```python
from build123d import *

# Parameters (mm, degrees)
F0_R           = 12.7
F1_DEPTH       = 7.9
F1_FACE_R      = 12.7
F2_DEPTH       = 3
F3_DEPTH       = 3
F4_R           = 5
F8_D           = 3.3
F8_CBORE_D     = 6
F8_CBORE_DEPTH = 3.3


# Not quite as in the source:
# - a feature names something its author has since deleted; it is built from what else it names


with BuildPart() as f1:
    # F0 (on Top) → F1 (new body)
    with BuildSketch(Plane.XY):
        with BuildLine():
            ThreePointArc((-82.519158721, -19.8666825891), (-82.3199649398, 11.4193737584), (-65.6162592679, 37.8739237785))
            Line((-65.6162592679, 37.8739237785), (-99.2088739193, 37.8739237785))
            ThreePointArc((-99.2088739193, 37.8739237785), (-117.1879721114, 26.6373104948), (-114.9666717313, 5.5523567478))
            Line((-114.9666717313, 5.5523567478), (-81.4747432756, -37.2867286205))
            Line((-81.4747432756, -37.2867286205), (-73.9695476283, -37.2867286205))
            Line((-73.9695476283, -37.2867286205), (-82.519158721, -19.8666825891))
        make_face()
        with Locations((-99.2088739193, 17.8719250206)):
            Circle(F0_R, mode=Mode.SUBTRACT)
    extrude(amount=-F1_DEPTH)



with BuildPart() as f1b:
    # F0 (on Top) → F1, piece 2 (new body)
    with BuildSketch(Plane.XY):
        with BuildLine():
            Line((86, -37.2867286205), (86, 37.8739237785))
            ThreePointArc((86, 37.8739237785), (76.5230858808, 21.4851908555), (70.8448413014, 3.4252903424))
            ThreePointArc((70.8448413014, 3.4252903424), (70.5487291916, -0.5692843065), (71.2877699379, -4.5060504646))
            ThreePointArc((71.2877699379, -4.5060504646), (77.4631412951, -21.4263167299), (86, -37.2867286205))
        make_face()
    extrude(amount=-F1_DEPTH)


with BuildPart() as f1_1:
    add(f1.part)

    add(f1b.part)  # F2 merges F1b
    # F0 (on Top) + F1_face (on face) → F2 (join)
    with BuildSketch(Plane.XY):
        with BuildLine():
            ThreePointArc((70.8448413014, 3.4252903424), (76.5230858808, 21.4851908555), (86, 37.8739237785))
            Line((86, 37.8739237785), (-65.6162592679, 37.8739237785))
            ThreePointArc((-65.6162592679, 37.8739237785), (-82.3199649398, 11.4193737584), (-82.519158721, -19.8666825891))
            Line((-82.519158721, -19.8666825891), (-73.9695476283, -37.2867286205))
            Line((-73.9695476283, -37.2867286205), (86, -37.2867286205))
            ThreePointArc((86, -37.2867286205), (77.4631412951, -21.4263167299), (71.2877699379, -4.5060504646))
            ThreePointArc((71.2877699379, -4.5060504646), (70.5487291916, -0.5692843065), (70.8448413014, 3.4252903424))
        make_face()
    with BuildSketch(Plane(origin=(-93.510683798, 7.7887517246, 0), x_dir=(1, 0, 0), z_dir=(0, 0, 1))):
        with BuildLine():
            ThreePointArc((10.9915250771, -27.6554343137), (11.1907188583, 3.6306220338), (27.8944245301, 30.0851720539))
            Line((27.8944245301, 30.0851720539), (-5.6981901212, 30.0851720539))
            ThreePointArc((-5.6981901212, 30.0851720539), (-23.6772883134, 18.8485587701), (-21.4559879333, -2.2363949769))
            Line((-21.4559879333, -2.2363949769), (12.0359405224, -45.0754803451))
            Line((12.0359405224, -45.0754803451), (19.5411361698, -45.0754803451))
            Line((19.5411361698, -45.0754803451), (10.9915250771, -27.6554343137))
        make_face()
        with Locations((-5.6981901212, 10.083173296)):
            Circle(F1_FACE_R, mode=Mode.SUBTRACT)
    extrude(amount=F2_DEPTH)

    # F4
    f4_edges = [f1_1.edges().sort_by_distance(p)[0] for p in [
        (-81.474743, -37.286729, -2.45),
    ]]
    fillet(f4_edges, radius=F4_R)


with BuildPart() as f3:
    # F0 (on Top) → F3 (new body)
    with BuildSketch(Plane.XY):
        with BuildLine():
            Line((86, -37.2867286205), (86, 37.8739237785))
            ThreePointArc((86, 37.8739237785), (76.5230858808, 21.4851908555), (70.8448413014, 3.4252903424))
            ThreePointArc((70.8448413014, 3.4252903424), (70.5487291916, -0.5692843065), (71.2877699379, -4.5060504646))
            ThreePointArc((71.2877699379, -4.5060504646), (77.4631412951, -21.4263167299), (86, -37.2867286205))
        make_face()
    extrude(amount=F3_DEPTH)


with BuildPart() as f1_2:
    add(f1_1.part)

    # F6: union F3
    add(f3.part)

    # F8 (through all)
    with Locations(Plane.XY.offset(3)):
        with Locations((-76.3588739193, 33.2139237785), (-113.9428039086, 24.5539237785), (-81.1954878403, -31.5067286205), (82.39, -23.6667286205), (82.39, 25.7039237785)):
            CounterBoreHole(F8_D / 2, F8_CBORE_D / 2, F8_CBORE_DEPTH)


solid = f1_2.part
```
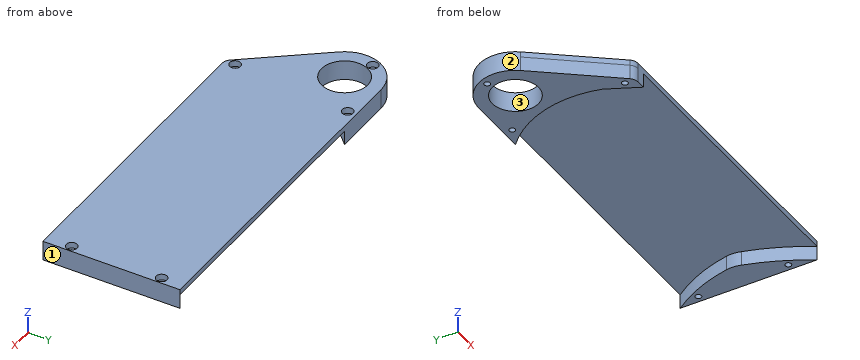
Geometry: final body of the model. Coordinates: model frame, mm. Face numbers are marked on the shaded views. Give positions to 0.01 mm unless a question says otherwise; leave off trailing zeros. Loops run counter-clockwise (first coordinate to the right, second up) from the corner with the lowest first, then second, coordinate; pieces in that order, holes last. Notation, with made-up numbers: (39, 89) - (45, 89) arc R21 ccw to (45, 103) - close; hole circle Ø9 at (32, 30.25). An arc over 180 degrees is marked (long way). Answer as CSV lines item,"result". Start each with the question number.
(1) Mould query, pull axis Y, two halves, no side actions, for the marked faces 1, 2 and 3. Classes: +Y half, -Y half, draft (parallel to the pull), parting line (faces both ways), or undercut.
(2) Section query C-C (y = -13). Output: boundary loops of the cut face in (x, z).
(3) Section query B-B (y = 14.5). Output: boundary loops of the cut face in (x, z), and give its area (3 significant figures).
(4) Ray query, line 1 along X through (y, z) = (15.5, -6.5); line 2 along Z through (x, y) = (-56.5, 22.5); line 3 along X through (y, z) = (-22.5, -1). Return the intervals inside material, ascending. Write a range as [from, to].
(5) Section query A-A (z = -5). Output: boundary loops of the cut face in (x, y).
(6) Pin query (flat end, axial travel): P1, Ø1.5, axis at y = -5.5, z = -4, coming from the -X side; P2, Ø1.8, axis at x = -80.5, y = -33, coming from the +Z side; P3, Ø1.5, axis at y = 24.5, z = -2.5, coming from the -X side. Return the tip coordinate at first contact, or that it passes through.
(7) Section query D-D (x = -58.5). Output: boundary loops of the cut face in (y, z), and give its area (3 significant figures).
Worked answers:
1,face 1,"draft"
1,face 2,"parting line"
1,face 3,"undercut"
2,outline,"(-100.46, -7.9) - (-83.99, -7.9) - (-83.99, 0) - (74.04, 0) - (74.04, -7.9) - (86, -7.9) - (86, 3) - (-100.46, 3) - close"
3,outline,"(-118.92, -7.9) - (-111.45, -7.9) - (-111.45, 3) - (-118.92, 3) - close; (-86.96, -7.9) - (-81.32, -7.9) - (-81.32, 0) - (73.81, 0) - (73.81, -7.9) - (86, -7.9) - (86, 3) - (-86.96, 3) - close"
3,area,"741 mm^2"
4,line 1,"x = [-119.07, -111.69], [-86.73, -80.96], [74.15, 86]"
4,line 2,"z = [0, 3]"
4,line 3,"x = [-93.04, -81.23], [77.95, 81.22], [83.56, 86]"
5,outline,"(-114.97, 5.55) - (-82.98, -35.37) arc R5 ccw to (-79.04, -37.29) - (-73.97, -37.29) - (-82.52, -19.87) arc R56.92 cw to (-65.62, 37.87) - (-99.21, 37.87) arc R20 ccw to start; (70.84, 3.43) arc R15.48 ccw to (71.29, -4.51) arc R125.34 ccw to (86, -37.29) - (86, 37.87) arc R86.36 ccw to start; hole circle Ø3.3 at (-113.94, 24.55); hole circle Ø25.4 at (-99.21, 17.87); hole circle Ø3.3 at (-81.2, -31.51); hole circle Ø3.3 at (-76.36, 33.21); hole circle Ø3.3 at (82.39, -23.67); hole circle Ø3.3 at (82.39, 25.7)"
6,P1,"stops at x = -106.91"
6,P2,"stops at z = -0.3"
6,P3,"stops at x = -118.33"
7,outline,"(-37.29, 0) - (37.87, 0) - (37.87, 3) - (-37.29, 3) - close"
7,area,"225 mm^2"
